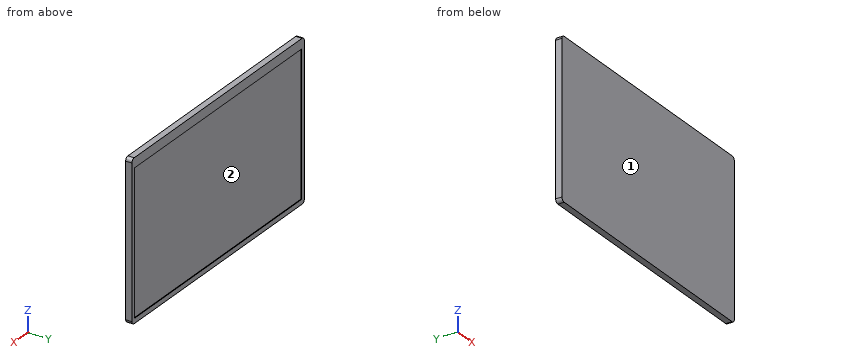
```python
from build123d import *

# Parameters (mm, degrees)
SKETCH_1_W          = 368
SKETCH_1_H          = 225
EXTRUDE_1_DEPTH     = 9
FILLET_1_R          = 5
SKETCH_2_W          = 356
SKETCH_2_H          = 204
CUT_EXTRUDE_1_DEPTH = 1


with BuildPart() as part:
    # 草图1 → 凸台-拉伸1 (new body)
    with BuildSketch(Plane(origin=(0, 0, 0), x_dir=(1, 0, 0), z_dir=(0, 1, 0))):
        Rectangle(SKETCH_1_W, SKETCH_1_H)
    extrude(amount=EXTRUDE_1_DEPTH)

    # 圆角1
    fillet_1_edges = [part.edges().sort_by_distance(p)[0] for p in [
        (-184, 4.5, -112.5),
        (184, 4.5, -112.5),
        (184, 4.5, 112.5),
        (-184, 4.5, 112.5),
    ]]
    fillet(fillet_1_edges, radius=FILLET_1_R)

    # 草图2 → 切除-拉伸1 (cut)
    with BuildSketch(Plane(origin=(0, 9, 0), x_dir=(1, 0, 0), z_dir=(0, 1, 0))):
        with Locations((0, 3.5)):
            Rectangle(SKETCH_2_W, SKETCH_2_H)
    extrude(amount=-CUT_EXTRUDE_1_DEPTH, mode=Mode.SUBTRACT)


solid = part.part
```
Part model, mm, in its own coordinate system. Face numbers are marked on the shaded views. Give positions to 0.01 mm unless a question says otherwise; leave off trailing zeros. Write each loop counter-clockwise with the first axis right and the second up, starting at its lowest first coordinate (ties: lowest second). Pieces come first, ordered by that corner, then holes. Notation, with made-up numbers: (74.25, 61.5) -> (91.25, 61.5) arc R11 ccw to (91.25, 77.5) -> close; hole circle Ø3 at (85, 67). An arc over 180 degrees is marked (long way). Put each result on its own line as item: value. Start each with the question number.
Item 1: Wall check: L1, parallel to Z at x = -30, y = 8.5; L2, parallel to Y at x = -61.5, z = 49. Give the ranges that are in metal, low to high. Write a range as [from, to].
Item 2: Pull direction X, two halves, no side cores. Call the marked faces 1 and 2: pulls with the +X half, pulls with the -X half, needs draft (parallel to the pull), parting line crosses it, or undercut.
Item 3: Pin check, flat tip, straight feed: pin 1 Ø10 at (x, z) = (-29.5, -53) entering from +Y. Stop position of the tip, or through.
Item 4: Cut at A-A (z = -8). List the corners of the cut face in (x, y), then the cut area to 3 significant figures.
Item 5: Cut at B-B (x = 70). List the corners of the cut face in (y, z).
Answer list:
1. L1: z = [-112.5, -105.5], [98.5, 112.5]
1. L2: y = [0, 8]
2. face 1: needs draft
2. face 2: undercut
3. pin 1: stops at y = 8
4. outline: (-184, 0) -> (184, 0) -> (184, 9) -> (178, 9) -> (178, 8) -> (-178, 8) -> (-178, 9) -> (-184, 9) -> close
4. area: 2,960 mm2
5. outline: (0, -112.5) -> (9, -112.5) -> (9, -105.5) -> (8, -105.5) -> (8, 98.5) -> (9, 98.5) -> (9, 112.5) -> (0, 112.5) -> close
